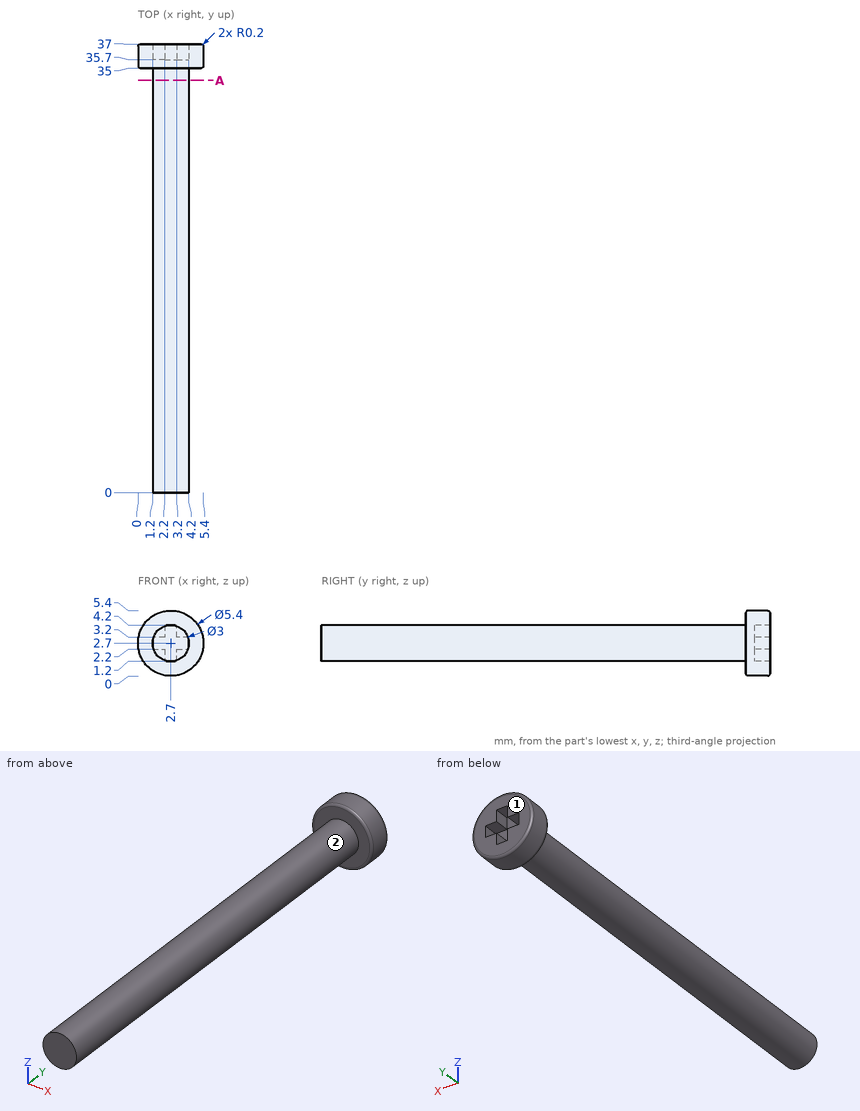
Source: three-view drawing plus pictorial views. Frame: mm from the lowest corner of the part. A direction names the side the tool comes from. Give positions to 0.01 mm unless a question says otherwise; leave off trailing zeros. Write each loop counter-clockwise with the first axis right and the second up, starting at its lowest first coordinate (ties: lowest second). Pieces come first, ordered by that corner, then holes.
(1) Access query for the marked faces 1 and 2. Directions: +Z, -Z, +X, -X, +Y, -Y. A direction counts if a zero-diameter tool reaches every point of the face in a straight line with its end or side. Return the directions, or none.
(2) First-contact query: P1, Ø0.5, axis at y = 36.5, z = 4, coming from the +X side; P2, Ø0.5, axis at x = 1.5, y = 36.5, coming from the +Z side; P3, Ø1, axis at y = 32, z = 3, coming from the -X side. Flat tips, straight axial feed; report the tip coordinate or a pass-through.
(3) Ray query, line 1 (Y direction, x = 1.6, z = 2.75); line 2 (Y direction, x = 1.7, z = 0.5); line 3 (X direction, y = 16.5, z = 2.25). Return the intervals inside material, ascending.
(4) Cut plane A-A, the plane y = 34. Return loops of the section in (x, z).
Values follow:
1. face 1: +Z, -Z, +X, -X, +Y
1. face 2: -Y
2. P1: stops at x = 5.19
2. P2: stops at z = 5.23
2. P3: stops at x = 1.2
3. line 1: y = 0 to 35.7
3. line 2: y = 35 to 37
3. line 3: x = 1.27 to 4.13
4. outline: circle Ø3 at (2.7, 2.7)
